Geometry check sheet. Reference: the model listing, model coordinates, mm. A direction names the side the tool comes from. Coordinates: 2 decimals unless noted, no trailing zeros. Loops run counter-clockwise (first coordinate to the right, second up) from the corner with the lowest first, then second, coordinate; pieces in that order, holes last. Notation, with made-up numbers: (85.25, 63) -> (100.25, 63) arc R34 ccw to (100.25, 102) -> close; hole circle Ø5 at (-10.75, 83.25). An arc over 180 degrees is marked (long way). Answer as a JSON object with one key per item and string values.
from build123d import *

# Parameters (mm, degrees)
SKETCH_W     = 15
SKETCH_H     = 15
PAD_DEPTH    = 7.5
POCKET_DEPTH = 7.501


with BuildPart() as part:
    # Sketch → Pad (new body)
    with BuildSketch(Plane.XY):
        with Locations((7.5, 7.5)):
            Rectangle(SKETCH_W, SKETCH_H)
    extrude(amount=PAD_DEPTH)

    # Sketch005 (on Face6 of Pad) → Pocket (cut, through all)
    with BuildSketch(Plane.XY.offset(7.5)):
        Polygon((1.75, 14), (13.25, 14), (7.5, 8.25), align=None)
        Polygon((1, 13.25), (6.75, 7.5), (1, 1.75), align=None)
        Polygon((1.75, 1), (7.5, 6.75), (13.25, 1), align=None)
        Polygon((8.25, 7.5), (14, 13.25), (14, 1.75), align=None)
    extrude(amount=-POCKET_DEPTH, mode=Mode.SUBTRACT)


solid = part.part
1. Mould release check, pull along Y, two halves, no side actions. Record for faces 3 (the face through (7, 0, 4)), 4 (the face through (7, 8, 0)), 5 (the face through (1, 7, 4)): released by +Y, released by -Y, zero draft, split by the parting line, or undercut.
Evaluation:
{"face 3": "released by -Y", "face 4": "zero draft", "face 5": "undercut"}
2. Section check B-B, the plane x = 12. Record the boundary of the cut face in (y, z), then the cut area to 3 significant figures.
Evaluation:
{"outline": "(0, 0) -> (1, 0) -> (1, 7.5) -> (0, 7.5) -> close; (2.25, 0) -> (3.75, 0) -> (3.75, 7.5) -> (2.25, 7.5) -> close; (11.25, 0) -> (12.75, 0) -> (12.75, 7.5) -> (11.25, 7.5) -> close; (14, 0) -> (15, 0) -> (15, 7.5) -> (14, 7.5) -> close", "area": "37.5 mm^2"}
3. Section check A-A, the plane y = 7.75. Record the boundary of the cut face in (x, z).
Evaluation:
{"outline": "(0, 0) -> (1, 0) -> (1, 7.5) -> (0, 7.5) -> close; (6.5, 0) -> (8.5, 0) -> (8.5, 7.5) -> (6.5, 7.5) -> close; (14, 0) -> (15, 0) -> (15, 7.5) -> (14, 7.5) -> close"}
4. Tool access check on faces 1 (the face through (8, 1, 4)), 2 (the face through (15, 7, 4)). Record the directions out of +Z, -Z, +X, -X, +Y, -Y that give a thin tool (end or side, any length) a straight path to the whole face; none if there is none.
Evaluation:
{"face 1": "+Z, -Z", "face 2": "+Z, -Z, +X, +Y, -Y"}
5. Section check C-C, the plane z = 2.75. Record the boundary of the cut face in (x, y).
Evaluation:
{"outline": "(0, 0) -> (15, 0) -> (15, 15) -> (0, 15) -> close; hole (1, 1.75) -> (6.75, 7.5) -> (1, 13.25) -> close; hole (1.75, 1) -> (13.25, 1) -> (7.5, 6.75) -> close; hole (1.75, 14) -> (7.5, 8.25) -> (13.25, 14) -> close; hole (8.25, 7.5) -> (14, 1.75) -> (14, 13.25) -> close"}
6. Section check D-D, the plane y = 10.25. Record the boundary of the cut face in (x, z).
Evaluation:
{"outline": "(0, 0) -> (1, 0) -> (1, 7.5) -> (0, 7.5) -> close; (4, 0) -> (5.5, 0) -> (5.5, 7.5) -> (4, 7.5) -> close; (9.5, 0) -> (11, 0) -> (11, 7.5) -> (9.5, 7.5) -> close; (14, 0) -> (15, 0) -> (15, 7.5) -> (14, 7.5) -> close"}
7. Thickness scan on probe 1 along X at (y, z) = (7.75, 7.25); probe 2 along X at (y, z) = (2.5, 2.25); probe 3 along X at (y, z) = (5.5, 6.25). Record the ranges inside material, lowest first. Write a range as from..to.
Evaluation:
{"probe 1": "x = 0..1, 6.5..8.5, 14..15", "probe 2": "x = 0..1, 1.75..3.25, 11.75..13.25, 14..15", "probe 3": "x = 0..1, 4.75..6.25, 8.75..10.25, 14..15"}
